```python
from build123d import *

# Parameters (mm, degrees)
SKETCH004_R          = 0.9
PAD_DEPTH            = 1.6
SKETCH007_W          = 10
SKETCH007_H          = 10.3
POCKET001_DEPTH      = 1.601
POCKET001_DEPTH_BACK = 1.601
POCKET_DEPTH         = 1.6
CHAMFER001_SIZE      = 0.4
SKETCH008_R          = 7.65
PAD001_DEPTH         = 5.6
CHAMFER_SIZE         = 0.4
SKETCH029_R          = 1.39
POCKET016_DEPTH      = 12.801
POCKET016_DEPTH_BACK = 9.201
CHAMFER002_SIZE      = 0.4
CHAMFER003_SIZE      = 0.3
CHAMFER004_SIZE      = 0.3
CHAMFER005_SIZE      = 0.4


with BuildPart() as part:
    # Sketch004 → Pad (new body, symmetric)
    with BuildSketch(Plane.XY.offset(-11.4)):
        with BuildLine():
            ThreePointArc((8.95, 10.9), (7.05, 12.8), (5.15, 10.9))
            Line((5.15, 9.2), (5.15, 10.9))
            Line((-7.75, 9.2), (5.15, 9.2))
            Line((-7.75, -5.1), (-7.75, 9.2))
            Line((-9.45, -5.1), (-7.75, -5.1))
            ThreePointArc((-9.45, -5.1), (-11.35, -7), (-9.45, -8.9))
            Line((-9.45, -8.9), (-7.75, -8.9))
            Line((-7.75, -8.9), (-7.75, -9.2))
            Line((9.25, -9.2), (-7.75, -9.2))
            Line((9.25, 9.2), (9.25, -9.2))
            Line((8.95, 9.2), (9.25, 9.2))
            Line((8.95, 10.9), (8.95, 9.2))
        make_face()
        with Locations((-9.45, -7)):
            Circle(SKETCH004_R, mode=Mode.SUBTRACT)
        with Locations((7.05, 10.9)):
            Circle(SKETCH004_R, mode=Mode.SUBTRACT)
    extrude(amount=PAD_DEPTH, both=True)

    # Sketch007 → Pocket001 (cut, two sides)
    with BuildSketch(Plane.XY.offset(-11.4)) as pocket001_sk:
        Rectangle(SKETCH007_W, SKETCH007_H)
    extrude(amount=-POCKET001_DEPTH, mode=Mode.SUBTRACT)
    extrude(pocket001_sk.sketch, amount=POCKET001_DEPTH_BACK, mode=Mode.SUBTRACT)

    # Sketch006 → Pocket (cut)
    with BuildSketch(Plane.XY.offset(-11.4)):
        with BuildLine():
            Line((8.45, 8), (8.45, -2.8))
            Line((11.05, -2.8), (8.45, -2.8))
            Line((11.05, -11), (11.05, -2.8))
            Line((4.45, -11), (11.05, -11))
            Line((4.45, -8.4), (4.45, -11))
            Line((-6.55, -8.4), (4.45, -8.4))
            Line((-6.55, -8.4), (-6.55, -8.9))
            Line((-6.55, -8.9), (-6.55, -9.2))
            Line((-6.55, -9.2), (-7.75, -9.2))
            Line((-7.75, -9.2), (-7.75, -8.9))
            Line((-9.65, -8.9), (-7.75, -8.9))
            ThreePointArc((-9.65, -5.1), (-11.55, -7), (-9.65, -8.9))
            Line((-9.65, -5.1), (-7.75, -5.1))
            Line((-7.75, -4.9), (-7.75, -5.1))
            Line((-7.75, -4.9), (-6.95, -4.9))
            Line((-6.95, 8.4), (-6.95, -4.9))
            Line((4.95, 8.4), (-6.95, 8.4))
            Line((4.95, 9.2), (4.95, 8.4))
            Line((4.95, 9.2), (5.15, 9.2))
            Line((5.15, 9.2), (5.15, 11.1))
            ThreePointArc((8.95, 11.1), (7.05, 13), (5.15, 11.1))
            Line((8.95, 11.1), (8.95, 9.2))
            Line((8.95, 9.2), (9.25, 9.2))
            Line((9.25, 8), (9.25, 9.2))
            Line((8.95, 8), (9.25, 8))
            Line((8.95, 8), (8.45, 8))
        make_face()
    extrude(amount=-POCKET_DEPTH, mode=Mode.SUBTRACT)

    # Chamfer001
    chamfer001_edges = [part.edges().sort_by_distance(p)[0] for p in [
        (-6.95, 1.75, -13),
        (-1, 8.4, -13),
        (8.45, 2.6, -13),
        (-1.05, -8.4, -13),
    ]]
    chamfer(chamfer001_edges, length=CHAMFER001_SIZE)

    # Sketch008 (on Face5 of Pocket001) → Pad001 (join)
    with BuildSketch(Plane.XY.offset(-9.8)):
        Circle(SKETCH008_R)
        Polygon((-4.4, 3.254487), (-3.254487, 4.4), (4.4, 4.4), (4.4, -4.4), (-4.4, -4.4), align=None, mode=Mode.SUBTRACT)
    extrude(amount=PAD001_DEPTH)

    # Chamfer
    chamfer_edges = [part.edges().sort_by_distance(p)[0] for p in [
        (4.4, 0, -4.2),
        (0.572756, 4.4, -4.2),
        (0, -4.4, -4.2),
        (-4.4, -0.572756, -4.2),
    ]]
    chamfer(chamfer_edges, length=CHAMFER_SIZE)

    # Sketch029 → Pocket016 (cut, two sides)
    with BuildSketch(Plane.XZ) as pocket016_sk:
        with Locations((0, -6.3)):
            Circle(SKETCH029_R)
    extrude(amount=-POCKET016_DEPTH, mode=Mode.SUBTRACT)
    extrude(pocket016_sk.sketch, amount=POCKET016_DEPTH_BACK, mode=Mode.SUBTRACT)

    # Chamfer002
    chamfer002_edges = [part.edges().sort_by_distance(p)[0] for p in [
        (-1.39, -7.522659, -6.3),
    ]]
    chamfer(chamfer002_edges, length=CHAMFER002_SIZE)

    # Chamfer003
    chamfer003_edges = [part.edges().sort_by_distance(p)[0] for p in [
        (-1.39, -4.4, -6.3),
    ]]
    chamfer(chamfer003_edges, length=CHAMFER003_SIZE)

    # Chamfer004
    chamfer004_edges = [part.edges().sort_by_distance(p)[0] for p in [
        (-1.39, 4.4, -6.3),
    ]]
    chamfer(chamfer004_edges, length=CHAMFER004_SIZE)

    # Chamfer005
    chamfer005_edges = [part.edges().sort_by_distance(p)[0] for p in [
        (-1.39, 7.522659, -6.3),
    ]]
    chamfer(chamfer005_edges, length=CHAMFER005_SIZE)


solid = part.part
```
Read the model definition and answer for the solid it produces. Units are mm, in the model's axes. A direction names the side the tool comes from. Round coordinates to 2 decimals unless told otherwise and drop trailing zeros. Write each loop counter-clockwise with the first axis right and the second up, starting at its lowest first coordinate (ties: lowest second). Pieces come first, ordered by that corner, then holes. Notation, with made-up numbers: (-1.75, 27.25) - (44.25, 27.25) arc R18 cw to (44.25, 49.25) - close; hole circle Ø1 at (5.25, 0.5). An arc over 180 degrees is marked (long way). Use CSV: the item, a comma, the result in double quotes.
Q1. A tool of negligible diameter and unlimited length cuts with its end or side. For faces 1 (the flat face through (4.95, 9, -12)), 2 (the flat face through (-7.75, 2, -11)), 3 (the flat face through (5, 0, -11)), 4 (the flat face through (8.95, 10, -11)), 5 (the flat face through (-4.4, -1, -7)), from which of +Z, -Z, +X, -X, +Y, -Y can it reach the whole face along a straight path? Write none if from no direction.
Values:
face 1,"-Z, +X, +Y, -Y"
face 2,"+Z, -Z, -X, +Y"
face 3,"-Z"
face 4,"+Z, -Z, +X, +Y"
face 5,"+Z, -Z"
Q2. Each of these flat-tipped pins is pushed along its axis until it touches: pin 1 Ø0.5 at (y, z) = (10, -10.5) entering from +X; pin 2 Ø6 at (x, y) = (0, 3.5) entering from -Z; pin 3 Ø4 at (y, z) = (7.5, -12) entering from -X. Where does it stop, or does it pass through?
Values:
pin 1,"stops at x = 8.95"
pin 2,"stops at z = -11.4"
pin 3,"stops at x = -7.75"
Q3. Find section A-A, the plane y = 0. Write down the section's boundary in (x, z).
Values:
outline,"(-7.75, -13) - (-7.35, -13) - (-6.95, -12.6) - (-6.95, -11.4) - (-5, -11.4) - (-5, -9.8) - (-4.4, -9.8) - (-4.4, -4.6) - (-4.8, -4.2) - (-7.65, -4.2) - (-7.65, -9.8) - (-7.75, -9.8) - close; (4.4, -9.8) - (5, -9.8) - (5, -11.4) - (8.45, -11.4) - (8.45, -12.6) - (8.85, -13) - (9.25, -13) - (9.25, -9.8) - (7.65, -9.8) - (7.65, -4.2) - (4.8, -4.2) - (4.4, -4.6) - close"
Q4. Straight lines are drawn through the part: line 1 along Y through (x, z) = (7.05, -10.7); line 2 along Y through (x, z) = (-9.45, -10.75); line 3 along X through (y, z) = (0.5, -10). For each, find the intervals that lie inside material, in ascending order.
Values:
line 1,"y = -9.2 to 10, 11.8 to 12.8"
line 2,"y = -8.9 to -7.9, -6.1 to -5.1"
line 3,"x = -7.75 to -5, 5 to 9.25"
Q5. Determine the mould class of faces 6 (the cylindrical face through (0.641, 5.957, -7.533)), 7 (the flat face through (-1, 9.2, -11)), 8 (the flat face through (-9, -8.9, -11)), 9 (the flat face through (6, 0, -11.4)) for opening direction Y: +Y half, -Y half, draft (parallel to the pull), parting line (faces both ways), or undercut.
Values:
face 6,"draft"
face 7,"+Y half"
face 8,"-Y half"
face 9,"undercut"
Q6. Find section D-D, the plane x = 0. Count the separate pieces of the cut face and the enclosed holes in it, then the cut area to 3 significant figures.
Values:
separate pieces,"4"
enclosed holes,"0"
area,"33.0 mm²"
Q7. Find section B-B, the plane x = 7.05. Write down the section's boundary in (y, z), then the cut area to 3 significant figures.
Values:
outline,"(-9.2, -11.4) - (10, -11.4) - (10, -9.8) - (2.97, -9.8) - (2.97, -4.2) - (-2.97, -4.2) - (-2.97, -9.8) - (-9.2, -9.8) - close; (11.8, -11.4) - (12.8, -11.4) - (12.8, -9.8) - (11.8, -9.8) - close"
area,"65.6 mm²"
Q8. Find section C-C, the plane z = -8.5. Write down the section's boundary in (x, y).
Values:
outline,"circle Ø15.3 at (0, 0); hole (-4.4, -4.4) - (4.4, -4.4) - (4.4, 4.4) - (-3.25, 4.4) - (-4.4, 3.25) - close"
